Geometry check sheet. Reference: the model listing, model coordinates, mm. A direction names the side the tool comes from. Give positions to 0.01 mm unless a question says otherwise; leave off trailing zeros. Write each loop counter-clockwise with the first axis right and the second up, starting at its lowest first coordinate (ties: lowest second). Pieces come first, ordered by that corner, then holes.
(1) Thickness scan on line 1 along Y through (x, z) = (-1.2, 2.5); line 2 along Y through (x, z) = (-0.3, -2); line 3 along Y through (x, z) = (0, 0.25). Record the ranges inside material, lowest first.
(2) Cross-section at B-B (y = -18.2). Record the boundary of the cut face in (x, z) (3 decimals), and give its area (4 significant figures).
(3) Depth check by flat-ended pin: P1, Ø1.8, axis at y = 8.8, z = 0, coming from the -X side. Enter the tip coordinate at first touch or a pass-through.
(4) Mould release check, pull along Z, two halves, no side actions. Record for faces 4 (the cylindrical face through (0, -16, 0)), 5 (the flat face through (-1, -24.75, 0)), 6 (the flat face through (0, 0, -3.25)): +Z half, -Z half, draft (parallel to the pull), parting line (faces both ways), or undercut.
(5) Tool access check on faces 1 (the flat face through (-1, 24.75, 0)), 2 (the flat face through (-1, 26, 0)), 3 (the cylindrical face through (0.38, -0.54, -2.44)). Record the directions out of +Z, -Z, +X, -X, +Y, -Y that give a thin tool (end or side, any length) a straight path to the whole face; none if there is none.
(6) Cross-section at A-A (x = -1.8). Record the boundary of the cut face in (y, z).
(7) Cross-section at D-D (y = 13.5). Record the boundary of the cut face in (x, z) (3 decimals), and give its area (4 significant figures).
(8) Cross-section at C-C (z = 0). Record the boundary of the cut face in (x, y) (3 decimals), and give its area (4 significant figures).
```python
from build123d import *

# Parameters (mm, degrees)
F0_W      = 52
F0_H      = 6.5
F1_DEPTH  = 0.625
F2_W      = 1.25
F2_H      = 6.5
F3_DEPTH  = 1.7
F4_R      = 0.25
F5_R      = 2.5
F6_DEPTH  = 1.25
F7_R      = 1
F8_DEPTH  = 1.25
F9_R      = 2.5
F10_DEPTH = 0.5


with BuildPart() as f1:
    # F0 (on Right) → F1 (new body, symmetric)
    with BuildSketch(Plane.YZ):
        Rectangle(F0_W, F0_H)
    extrude(amount=F1_DEPTH, both=True)

    # F2 (on face) → F3 (join)
    with BuildSketch(Plane(origin=(-0.625, 0, 0), x_dir=(0, -1, 0), z_dir=(-1, 0, 0))):
        with Locations((-25.375, 0)):
            Rectangle(F2_W, F2_H)
        with Locations((25.375, 0)):
            Rectangle(F2_W, F2_H)
    extrude(amount=F3_DEPTH)

    # F4
    f4_edges = [f1.edges().sort_by_distance(p)[0] for p in [
        (-0.85, -26, 3.25),
        (-0.85, -26, -3.25),
        (-0.85, 26, 3.25),
        (-0.85, 26, -3.25),
    ]]
    fillet(f4_edges, radius=F4_R)

    # F5 (on face) → F6 (cut, through all)
    with BuildSketch(Plane.YZ.offset(0.625)):
        with Locations((-13.5, 0)):
            Circle(F5_R)
        with Locations((13.5, 0)):
            Circle(F5_R)
    extrude(amount=-F6_DEPTH, mode=Mode.SUBTRACT)

    # F7 (on face) → F8 (cut, through all)
    with BuildSketch(Plane(origin=(-0.625, 0, 0), x_dir=(0, -1, 0), z_dir=(-1, 0, 0))):
        with Locations((-8.8, 0)):
            Circle(F7_R)
        with Locations((18.2, 0)):
            Circle(F7_R)
    extrude(amount=-F8_DEPTH, mode=Mode.SUBTRACT)

    # F9 (on face) → F10 (cut)
    with BuildSketch(Plane.YZ.offset(0.625)):
        Circle(F9_R)
    extrude(amount=-F10_DEPTH, mode=Mode.SUBTRACT)


solid = f1.part
```
Reply:
1. line 1: y = -26 to -24.75, 24.75 to 26
1. line 2: y = -26 to -15, -12 to 12, 15 to 26
1. line 3: y = -26 to -19.17, -17.23 to -15.99, -11.01 to 7.83, 9.77 to 11.01, 15.99 to 26
2. outline: (-0.625, -3.25) - (0.625, -3.25) - (0.625, -1) - (-0.625, -1) - close; (-0.625, 1) - (0.625, 1) - (0.625, 3.25) - (-0.625, 3.25) - close
2. area: 5.625 mm2
3. P1: passes through
4. face 4: undercut
4. face 5: draft
4. face 6: -Z half
5. face 1: +Z, -Z, -X
5. face 2: +Z, -Z, +X, -X, +Y
5. face 3: +X
6. outline: (-26, -3) arc R0.25 ccw to (-25.75, -3.25) - (-24.75, -3.25) - (-24.75, 3.25) - (-25.75, 3.25) arc R0.25 ccw to (-26, 3) - close; (24.75, -3.25) - (25.75, -3.25) arc R0.25 ccw to (26, -3) - (26, 3) arc R0.25 ccw to (25.75, 3.25) - (24.75, 3.25) - close
7. outline: (-0.625, -3.25) - (0.625, -3.25) - (0.625, -2.5) - (-0.625, -2.5) - close; (-0.625, 2.5) - (0.625, 2.5) - (0.625, 3.25) - (-0.625, 3.25) - close
7. area: 1.875 mm2
8. outline: (-2.325, -26) - (0.625, -26) - (0.625, -19.2) - (-0.625, -19.2) - (-0.625, -24.75) - (-2.325, -24.75) - close; (-2.325, 24.75) - (-0.625, 24.75) - (-0.625, 16) - (0.625, 16) - (0.625, 26) - (-2.325, 26) - close; (-0.625, -17.2) - (0.625, -17.2) - (0.625, -16) - (-0.625, -16) - close; (-0.625, -11) - (0.625, -11) - (0.625, -2.5) - (0.125, -2.5) - (0.125, 2.5) - (0.625, 2.5) - (0.625, 7.8) - (-0.625, 7.8) - close; (-0.625, 9.8) - (0.625, 9.8) - (0.625, 11) - (-0.625, 11) - close
8. area: 49.25 mm2
